Source: CAD feature listing. Evaluate the final solid. Frame: model axes, mm. Face numbers are marked on the shaded views. Give positions to 0.01 mm unless a question says otherwise; leave off trailing zeros. Order: outer loops, then holes, each group sorted by start corner. A loop starts at its lowest first (then second) coordinate and runs counter-clockwise, first axis right, second up.
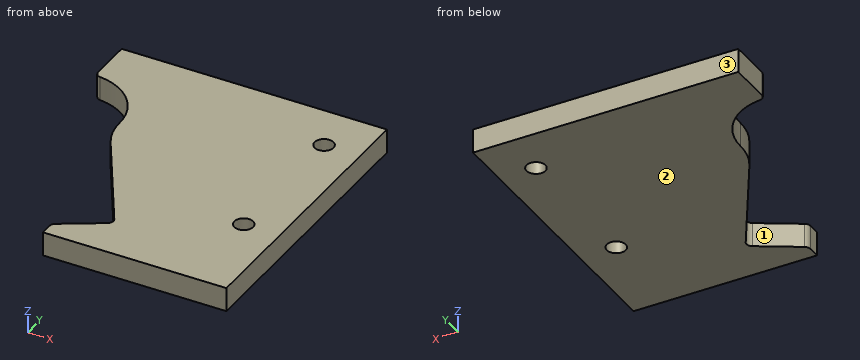
from build123d import *

# Parameters (mm, degrees)
SKETCH1_R           = 2.4892
BOSS_EXTRUDE1_DEPTH = 3.175
FILLET1_R           = 1.5875


with BuildPart() as part:
    # Sketch1 → Boss-Extrude1 (new, symmetric)
    with BuildSketch(Plane.XY):
        with BuildLine():
            Line((69.85, 27.3812), (69.85, -48.8188))
            Line((69.85, -48.8188), (21.576606, -48.8188))
            Line((21.576606, -48.8188), (21.576606, -44.762860113))
            Line((21.576606, -44.762860113), (34.055016522, -37.397839205))
            Line((34.055016522, -37.397839205), (16.883960941, -8.3052564))
            ThreePointArc((16.883960941, -8.3052564), (15.225065006, -4.359245427), (14.68076155, -0.11346257))
            ThreePointArc((14.68076155, -0.11346257), (10.421213944, 10.340983192), (0, 14.6812))
            Line((0, 14.6812), (0, 27.3812))
            Line((0, 27.3812), (69.85, 27.3812))
        make_face()
        with Locations((60.325, 14.6812)):
            Circle(SKETCH1_R, mode=Mode.SUBTRACT)
        with Locations((60.325, -23.4188)):
            Circle(SKETCH1_R, mode=Mode.SUBTRACT)
    extrude(amount=BOSS_EXTRUDE1_DEPTH, both=True)

    # Fillet1
    fillet1_edges = [part.edges().sort_by_distance(p)[0] for p in [
        (21.576606, -44.762860113, 0),
        (34.055016522, -37.397839205, 0),
        (0, 14.6812, 0),
    ]]
    fillet(fillet1_edges, radius=FILLET1_R)


solid = part.part
1) Section query A-A on x = 24. Output: boundary loops of the cut face in (y, z) (3 decimals).
Checks:
outline: (-48.819, -3.175) - (-43.333, -3.175) - (-43.333, 3.175) - (-48.819, 3.175) - close; (-20.362, -3.175) - (27.381, -3.175) - (27.381, 3.175) - (-20.362, 3.175) - close
2) Section query C-C on y = 6. Output: boundary loops of the cut face in (x, z) (3 decimals), and give its area (3 significant figures).
Checks:
outline: (13.399, -3.175) - (69.85, -3.175) - (69.85, 3.175) - (13.399, 3.175) - close
area: 358 mm2
3) Section query B-B on z = 0.5. State how many separate pieces and enclosed holes the cut face has, and give its area (3 significant figures).
Checks:
separate pieces: 1
enclosed holes: 2
area: 3,950 mm2
4) First-contact query: pin 1 Ø3.5 at (y, z) = (-48, 1) entering from -X; pin 2 Ø6.5 at (x, y) = (60.32, -23.42) entering from +Z (3 decimals). Flat tips, straight axial feed; report the tip coordinate or a pass-through.
Checks:
pin 1: stops at x = 21.58
pin 2: stops at z = 3.175
5) Section query D-D on y = -35. Output: boundary loops of the cut face in (x, z) (3 decimals).
Checks:
outline: (32.64, -3.175) - (69.85, -3.175) - (69.85, 3.175) - (32.64, 3.175) - close
6) Pull-direction query (Y, two-part tool) for the marked faces 1, 2 and 3; classes: +Y half, -Y half, draft (parallel to the pull), parting line (faces both ways), or undercut.
Checks:
face 1: undercut
face 2: draft
face 3: +Y half
7) Ray query, L1, parallel to Y at x = 60, z = -1.25; L2, parallel to Y at x = 59, z = 1.5; L3, parallel to X at y = -37, z = 1.5. Return the intervals inside material, ascending.
Checks:
L1: y = -48.82 to -25.89, -20.95 to 12.21, 17.15 to 27.38
L2: y = -48.82 to -25.53, -21.31 to 12.57, 16.79 to 27.38
L3: x = 33.46 to 69.85
